from build123d import *

# Parameters (mm, degrees)
EXTRUDE_1_DEPTH = 484.6


with BuildPart() as part:
    # Эскиз1 → Бобышка-Вытянуть1 (new body)
    with BuildSketch(Plane.XY):
        with BuildLine():
            Line((-12, 15), (12, 15))
            ThreePointArc((12, 15), (14.121320344, 14.121320344), (15, 12))
            Line((15, 12), (15, -12))
            ThreePointArc((15, -12), (14.121320344, -14.121320344), (12, -15))
            Line((12, -15), (-12, -15))
            ThreePointArc((-12, -15), (-14.121320344, -14.121320344), (-15, -12))
            Line((-15, -12), (-15, 12))
            ThreePointArc((-15, 12), (-14.121320344, 14.121320344), (-12, 15))
        make_face()
        with BuildLine():
            Line((-11, 13), (11, 13))
            ThreePointArc((11, 13), (12.414213562, 12.414213562), (13, 11))
            Line((13, 11), (13, -11))
            ThreePointArc((13, -11), (12.414213562, -12.414213562), (11, -13))
            Line((11, -13), (-11, -13))
            ThreePointArc((-11, -13), (-12.414213562, -12.414213562), (-13, -11))
            Line((-13, -11), (-13, 11))
            ThreePointArc((-13, 11), (-12.414213562, 12.414213562), (-11, 13))
        make_face(mode=Mode.SUBTRACT)
    extrude(amount=EXTRUDE_1_DEPTH)

    # Зеркальное отражение1: part across plane


with BuildPart() as part_1:
    add(part.part)
    add(part.part.mirror(Plane(origin=(-12, -12, 0), x_dir=(1, 0, 0), z_dir=(0, 0, 1))))


solid = part_1.part
The listing builds one solid part. Answer for the finished solid, in the listing's coordinates (mm). A direction names the side the tool comes from. Give positions to 0.01 mm unless a question says otherwise; leave off trailing zeros. Loops run counter-clockwise (first coordinate to the right, second up) from the corner with the lowest first, then second, coordinate; pieces in that order, holes last. Notation, with made-up numbers: (36, 63) - (69, 63) arc R26 cw to (69, 102) - close; hole circle Ø11 at (-36.5, 39.25). An arc over 180 degrees is marked (long way). Use one line per item in the form item = value.
1. The mould has two halves that part along X. Classify faces 3 (the face through (0, 13, 7)), 4 (the face through (15, 0, 7)), 5 (the face through (0, -15, 7)): pulls with the +X half, pulls with the -X half, needs draft (parallel to the pull), parting line crosses it, or undercut.
Calculated:
face_3 = undercut
face_4 = pulls with the +X half
face_5 = needs draft
2. Section A-A on y = -0.5 is taken. Give the vertices of the cut face in (x, z).
Calculated:
outline = (-15, -484.6) - (-13, -484.6) - (-13, 484.6) - (-15, 484.6) - close; (13, -484.6) - (15, -484.6) - (15, 484.6) - (13, 484.6) - close
3. Find the intervals of material crossed by line 1 along X through (y, z) = (-10, -303); line 2 along Y through (x, z) = (11.75, -69), in increasing order. Write a range as [from, to].
Calculated:
line_1 = [-15, -13], [13, 15]
line_2 = [-15, -12.85], [12.85, 15]
4. Which of the six approach directions +Z, -Z, +X, -X, +Y, -Y give full straight-line access (tool end or side, diameter ignored) to faces 1 (the face through (-13, 0, 7)), 2 (the face through (14, 0, 484.6))?
Calculated:
face_1 = +Z, -Z
face_2 = +Z, +X, -X, +Y, -Y
5. Section C-C on z = 118 is taken. Give the vertices of the cut face in (x, y).
Calculated:
outline = (-15, -12) arc R3 ccw to (-12, -15) - (12, -15) arc R3 ccw to (15, -12) - (15, 12) arc R3 ccw to (12, 15) - (-12, 15) arc R3 ccw to (-15, 12) - close; hole (-13, -11) arc R2 ccw to (-11, -13) - (11, -13) arc R2 ccw to (13, -11) - (13, 11) arc R2 ccw to (11, 13) - (-11, 13) arc R2 ccw to (-13, 11) - close
